Source: CAD feature listing. Evaluate the final solid. Frame: model axes, mm. Face numbers are marked on the shaded views. A direction names the side the tool comes from. Coordinates: 2 decimals unless noted, no trailing zeros. Order: outer loops, then holes, each group sorted by start corner. A loop starts at its lowest first (then second) coordinate and runs counter-clockwise, first axis right, second up.
```python
from build123d import *

# Parameters (mm, degrees)
SKIZZE1_R                       = 20
SKIZZE1_R_2                     = 7
AUFSATZ_LINEAR_AUSTRAGEN1_DEPTH = 5.5
SCHNITT_LINEAR_AUSTRAGEN1_DEPTH = 4
SCHNITT_LINEAR_AUSTRAGEN2_REACH = 7.5
SKIZZE3_R                       = 1.25
SCHNITT_LINEAR_AUSTRAGEN3_REACH = 3.5
SKIZZE4_R                       = 0.75
VERRUNDUNG1_R                   = 1


with BuildPart() as part:
    # Skizze1 → Aufsatz-Linear austragen1 (new body)
    with BuildSketch(Plane.XY):
        Circle(SKIZZE1_R)
        Circle(SKIZZE1_R_2, mode=Mode.SUBTRACT)
    extrude(amount=AUFSATZ_LINEAR_AUSTRAGEN1_DEPTH)

    # Skizze2 → Schnitt-Linear austragen1 (cut)
    with BuildSketch(Plane.XY.offset(5.5)):
        with BuildLine():
            Line((-4.630064794, -5.25), (-12.165525061, -5.25))
            ThreePointArc((-12.165525061, -5.25), (0, -13.25), (12.165525061, -5.25))
            Line((12.165525061, -5.25), (4.630064794, -5.25))
            ThreePointArc((4.630064794, -5.25), (0, -7), (-4.630064794, -5.25))
        make_face()
        with BuildLine():
            ThreePointArc((-12.165525061, 5.25), (-13.25, 0), (-12.165525061, -5.25))
            Line((-12.165525061, -5.25), (-4.630064794, -5.25))
            ThreePointArc((-4.630064794, -5.25), (-7, 0), (-4.630064794, 5.25))
            Line((-4.630064794, 5.25), (-12.165525061, 5.25))
        make_face()
        with BuildLine():
            Line((4.630064794, -5.25), (12.165525061, -5.25))
            ThreePointArc((12.165525061, -5.25), (12.976049226, -2.680419085), (13.25, 0))
            ThreePointArc((13.25, 0), (12.976049226, 2.680419085), (12.165525061, 5.25))
            Line((12.165525061, 5.25), (4.630064794, 5.25))
            ThreePointArc((4.630064794, 5.25), (6.380064794, 2.880064794), (7, 0))
            ThreePointArc((7, 0), (6.380064794, -2.880064794), (4.630064794, -5.25))
        make_face()
        with BuildLine():
            ThreePointArc((12.165525061, 5.25), (0, 13.25), (-12.165525061, 5.25))
            Line((-12.165525061, 5.25), (-4.630064794, 5.25))
            ThreePointArc((-4.630064794, 5.25), (0, 7), (4.630064794, 5.25))
            Line((4.630064794, 5.25), (12.165525061, 5.25))
        make_face()
        with BuildLine():
            Line((-15.25, 5.25), (-15.25, -5.25))
            Line((-15.25, -5.25), (-12.165525061, -5.25))
            ThreePointArc((-12.165525061, -5.25), (-13.25, 0), (-12.165525061, 5.25))
            Line((-12.165525061, 5.25), (-15.25, 5.25))
        make_face()
        with BuildLine():
            ThreePointArc((13.25, 0), (12.976049226, -2.680419085), (12.165525061, -5.25))
            Line((12.165525061, -5.25), (15.25, -5.25))
            Line((15.25, -5.25), (15.25, 5.25))
            Line((15.25, 5.25), (12.165525061, 5.25))
            ThreePointArc((12.165525061, 5.25), (12.976049226, 2.680419085), (13.25, 0))
        make_face()
    extrude(amount=-SCHNITT_LINEAR_AUSTRAGEN1_DEPTH, mode=Mode.SUBTRACT)

    # Skizze3 → Schnitt-Linear austragen2 (cut, up to next)
    with BuildSketch(Plane.XY.offset(5.5), mode=Mode.PRIVATE) as schnitt_linear_austragen2_sk1:
        with Locations((13, 0)):
            Circle(SKIZZE3_R)
    schnitt_linear_austragen2_tool1 = extrude(schnitt_linear_austragen2_sk1.sketch, amount=-SCHNITT_LINEAR_AUSTRAGEN2_REACH, mode=Mode.PRIVATE) & part.part
    add(schnitt_linear_austragen2_tool1.solids().sort_by_distance((13, 0, 5.5))[0], mode=Mode.SUBTRACT)
    # Skizze3 → Schnitt-Linear austragen2 (cut, up to next)
    with BuildSketch(Plane.XY.offset(5.5), mode=Mode.PRIVATE) as schnitt_linear_austragen2_sk2:
        with Locations((-13, 0)):
            Circle(SKIZZE3_R)
    schnitt_linear_austragen2_tool2 = extrude(schnitt_linear_austragen2_sk2.sketch, amount=-SCHNITT_LINEAR_AUSTRAGEN2_REACH, mode=Mode.PRIVATE) & part.part
    add(schnitt_linear_austragen2_tool2.solids().sort_by_distance((-13, 0, 5.5))[0], mode=Mode.SUBTRACT)

    # Skizze4 → Schnitt-Linear austragen3 (cut, up to next)
    with BuildSketch(Plane.XY.offset(1.5), mode=Mode.PRIVATE) as schnitt_linear_austragen3_sk1:
        with Locations((0, -7)):
            Circle(SKIZZE4_R)
    schnitt_linear_austragen3_tool1 = extrude(schnitt_linear_austragen3_sk1.sketch, amount=-SCHNITT_LINEAR_AUSTRAGEN3_REACH, mode=Mode.PRIVATE) & part.part
    add(schnitt_linear_austragen3_tool1.solids().sort_by_distance((0, -7, 1.5))[0], mode=Mode.SUBTRACT)

    # Verrundung1
    verrundung1_edges = [part.edges().sort_by_distance(p)[0] for p in [
        (-0.748923015, -6.959821429, 0.75),
        (0.748923015, -6.959821429, 0.75),
    ]]
    fillet(verrundung1_edges, radius=VERRUNDUNG1_R)


solid = part.part
```
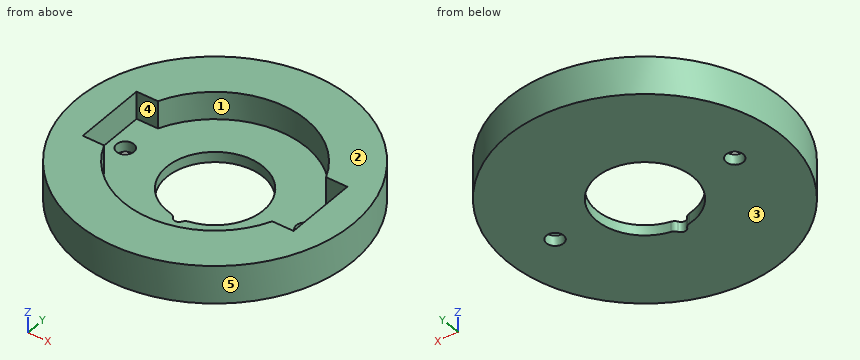
Q1. Section query D-D on x = -13.5. Output: boundary loops of the cut face in (y, z).
Solutions:
outline: (-14.76, 0) - (-1.15, 0) - (-1.15, 1.5) - (-5.25, 1.5) - (-5.25, 5.5) - (-14.76, 5.5) - close; (1.15, 0) - (14.76, 0) - (14.76, 5.5) - (5.25, 5.5) - (5.25, 1.5) - (1.15, 1.5) - close
Q2. Set-up query: the marked faces 1 and 2. Return all of +Z, -Z, +X, -X, +Y, -Y with unobstructed straight access to the full face (end or side cutting, diameter ignored); none if empty.
Solutions:
face 1: +Z
face 2: +Z, +X, -X, +Y, -Y
Q3. Section query B-B on y = 0. Output: boundary loops of the cut face in (x, z), plus the area to 3 significant figures.
Solutions:
outline: (-20, 0) - (-14.25, 0) - (-14.25, 1.5) - (-15.25, 1.5) - (-15.25, 5.5) - (-20, 5.5) - close; (-11.75, 0) - (-7, 0) - (-7, 1.5) - (-11.75, 1.5) - close; (7, 0) - (11.75, 0) - (11.75, 1.5) - (7, 1.5) - close; (14.25, 0) - (20, 0) - (20, 5.5) - (15.25, 5.5) - (15.25, 1.5) - (14.25, 1.5) - close
area: 69.5 mm2
Q4. Pin query (flat end, axial travel): P1, Ø3, axis at x = 10, z = 2.5, coming from the -Y side; P2, Ø2.5, axis at x = 14.5, z = 4, coming from the +Y side; P3, Ø2.5, axis at x = -13, z = 3, coming from the -Y side. Return the tip coordinate at first contact, or that it passes through.
Solutions:
P1: stops at y = -18.1
P2: stops at y = 14.98
P3: stops at y = -16.18
Q5. Material intervals for line 1 along X through (y, z) = (-0.5, 4); line 2 along X through (y, z) = (-0.5, 1.45); line 3 along Z through (x, y) = (-11.5, 3.5), sorted ascending.
Solutions:
line 1: x = -19.99 to -15.25, 15.25 to 19.99
line 2: x = -19.99 to -14.15, -11.85 to -6.98, 6.98 to 11.85, 14.15 to 19.99
line 3: z = 0 to 1.5
Q6. Section query A-A on x = 0. Output: boundary loops of the cut face in (y, z).
Solutions:
outline: (-20, 0) - (-7.75, 0) - (-7.75, 1.5) - (-13.25, 1.5) - (-13.25, 5.5) - (-20, 5.5) - close; (7, 0) - (20, 0) - (20, 5.5) - (13.25, 5.5) - (13.25, 1.5) - (7, 1.5) - close
Q7. Section query C-C on z = 4.3. Output: boundary loops of the cut face in (x, y), plus the area to 3 significant figures.
Solutions:
outline: circle Ø40 at (0, 0); hole (-15.25, -5.25) - (-12.17, -5.25) arc R13.25 ccw to (12.17, -5.25) - (15.25, -5.25) - (15.25, 5.25) - (12.17, 5.25) arc R13.25 ccw to (-12.17, 5.25) - (-15.25, 5.25) - close
area: 656 mm2
Q8. Pull-direction query (X, two-part tool) for the marked faces 3, 4 and 5; classes: pulls with the +X half, pulls with the -X half, needs draft (parallel to the pull), parting line crosses it, or undercut.
Solutions:
face 3: needs draft
face 4: undercut
face 5: parting line crosses it
